Work out the finished part from the listing and answer in its coordinate system (mm). Face numbers are marked on the shaded views. Give positions to 0.01 mm unless a question says otherwise; leave off trailing zeros. Write each loop counter-clockwise with the first axis right and the second up, starting at its lowest first coordinate (ties: lowest second). Pieces come first, ordered by that corner, then holes.
1) Find section C-C (y = -33). Determine the outline of the cut face in (x, z).
2) Given pin 1 Ø3 at (x, y) = (-83.5, -14.5) entering from -Z; pin 2 Ø0.8 at (x, z) = (-30, -0.5) entering from -Y; pin 3 Ø0.5 at (y, z) = (-12.5, -0.5) entering from -X, each flat-ended and moving along its own axis, determine where each tip first touches the part or whether it passes through.
3) Find section A-A (y = -21.5). Determine the outline of the cut face in (x, z), plus the area to 3 significant figures.
4) Find section B-B (x = -116.5). Determine the outline of the cut face in (y, z).
5) Straight lines are drawn through the part: probe 1 along X at (y, z) = (-33, -0.25); probe 2 along Y at (x, z) = (-119.5, 6); probe 3 along Z at (x, y) = (-5, -27). For each, find the intervals that lie inside material, in ascending order.
6) Determine the mould class of the marked faces 1 and 2 for opening direction X: pulls with the +X half, pulls with the -X half, needs draft (parallel to the pull), parting line crosses it, or undercut.
7) Find section D-D (x = -52). Determine the outline of the cut face in (y, z).
```python
from build123d import *

# Parameters (mm, degrees)
SKETCH1_W               = 129.063503861
SKETCH1_H               = 57.862502499
BOSS_EXTRUDE1_DEPTH     = 5
SKETCH2_W               = 36.260872389
SKETCH2_H               = 45.239555314
SKETCH2_W_2             = 34.782772322
SKETCH2_H_2             = 43.550253841
BOSS_EXTRUDE2_DEPTH     = 1
SKETCH3_R               = 3.560103521
BOSS_EXTRUDE3_DEPTH     = 1
CUT_EXTRUDE2_DEPTH      = 0.5
CUT_EXTRUDE3_DEPTH      = 0.5
SKETCH11_W              = 140.269028905
SKETCH11_H              = 63.169878757
BOSS_EXTRUDE4_DEPTH     = 2
CUT_EXTRUDE11_DEPTH     = 146.740563875
CUT_EXTRUDE12_DEPTH     = 149.974025726
CUT_EXTRUDE15_DEPTH     = 149.535595308
CUT_EXTRUDE18_DEPTH     = 149.974025726
CUT_EXTRUDE20_START     = -22.544046022
CUT_EXTRUDE20_OUTLINE_W = 10.649091721
CUT_EXTRUDE20_OUTLINE_H = 19.66096559
CUT_EXTRUDE20_DEPTH     = 22.544046022


# Read off the part's stored shape, not the designer's step: Cut-Extrude20
with BuildPart() as part:
    # Sketch1 → Boss-Extrude1 (new body)
    with BuildSketch(Plane.XY):
        with Locations((-61.962065286, -16.351878859)):
            Rectangle(SKETCH1_W, SKETCH1_H)
    extrude(amount=BOSS_EXTRUDE1_DEPTH)

    # Sketch2 → Boss-Extrude2 (add)
    with BuildSketch(Plane(origin=(0, 0, 0), x_dir=(-1, 0, 0), z_dir=(0, 0, -1))):
        with Locations((32.418116178, -15.92763049)):
            Rectangle(SKETCH2_W, SKETCH2_H)
        with Locations((32.418116178, -15.92763049)):
            Rectangle(SKETCH2_W_2, SKETCH2_H_2, mode=Mode.SUBTRACT)
    extrude(amount=BOSS_EXTRUDE2_DEPTH)

    # Sketch3 → Boss-Extrude3 (add)
    with BuildSketch(Plane(origin=(0, 0, 0), x_dir=(-1, 0, 0), z_dir=(0, 0, -1))):
        with Locations((5.84715491, -15.809376146)):
            Circle(SKETCH3_R)
    extrude(amount=BOSS_EXTRUDE3_DEPTH)

    # Sketch4 → Cut-Extrude2 (cut)
    with BuildSketch(Plane(origin=(0, 0, -1), x_dir=(-1, 0, 0), z_dir=(0, 0, -1))):
        with BuildLine():
            Line((7.498244586, -13.503730374), (7.429945817, -14.22683494))
            ThreePointArc((7.429945817, -14.22683494), (3.750240849, -15.79486572), (7.319195969, -17.600830429))
            Line((7.319195969, -17.600830429), (7.313770936, -18.341402976))
            ThreePointArc((7.313770936, -18.341402976), (3.134365244, -15.759677296), (7.498244586, -13.503730374))
        make_face()
    extrude(amount=-CUT_EXTRUDE2_DEPTH, mode=Mode.SUBTRACT)

    # Sketch5 → Cut-Extrude3 (cut)
    with BuildSketch(Plane(origin=(0, 0, -1), x_dir=(-1, 0, 0), z_dir=(0, 0, -1))):
        with BuildLine():
            Line((8.340052895, -15.49291333), (5.46397868, -15.438165983))
            ThreePointArc((5.46397868, -15.438165983), (5.066360432, -15.835784231), (5.46397868, -16.233402479))
            Line((5.46397868, -16.233402479), (8.340052895, -16.178655131))
            ThreePointArc((8.340052895, -16.178655131), (8.682923796, -15.835784231), (8.340052895, -15.49291333))
        make_face()
    extrude(amount=-CUT_EXTRUDE3_DEPTH, mode=Mode.SUBTRACT)

    # Sketch11 → Boss-Extrude4 (add)
    with BuildSketch(Plane.XY.offset(5)):
        with Locations((-64.601623086, -16.772300036)):
            Rectangle(SKETCH11_W, SKETCH11_H)
    extrude(amount=BOSS_EXTRUDE4_DEPTH)

    # Sketch12 → Cut-Extrude11 (cut, through all)
    with BuildSketch(Plane(origin=(2.569686645, 0, 0), x_dir=(0, 0, -1), z_dir=(1, 0, 0))):
        Polygon((-5.049502584, 12.555506791), (1.376837193, 8.637811028), (1.49491418, 17.884962826), align=None)
    extrude(amount=-CUT_EXTRUDE11_DEPTH, mode=Mode.SUBTRACT)

    # Sketch13 → Cut-Extrude12 (cut, through all)
    with BuildSketch(Plane(origin=(0, 14.812639343, 0), x_dir=(1, 0, 0), z_dir=(0, 1, 0))):
        Polygon((-126.405113906, -5), (-129.311029141, 1.46898876), (-122.374079844, 2.014276014), align=None)
    extrude(amount=-CUT_EXTRUDE12_DEPTH, mode=Mode.SUBTRACT)

    # Sketch14 → Cut-Extrude15 (cut, through all)
    with BuildSketch(Plane.ZY.offset(134.736137539)):
        Polygon((5, -45.234938719), (-1.330755584, -41.178219973), (-1.62330097, -49.506029315), align=None)
    extrude(amount=-CUT_EXTRUDE15_DEPTH, mode=Mode.SUBTRACT)

    # Sketch15 → Cut-Extrude18 (cut, through all)
    with BuildSketch(Plane(origin=(0, -48.357239414, 0), x_dir=(-1, 0, 0), z_dir=(0, -1, 0))):
        Polygon((-2.559600043, -5), (1.778800488, 1.23954643), (-4.071250311, 1.127548689), align=None)
    extrude(amount=-CUT_EXTRUDE18_DEPTH, mode=Mode.SUBTRACT)

    # Cut-Extrude20 outline → Cut-Extrude20 (cut)
    with BuildSketch(Plane(origin=(-92.862199247, 0, -53.366974362), x_dir=(-0.49826909719441087, 0, 0.8670224372996739), z_dir=(-0.8670224372996738, 0, -0.4982690971944108)).offset(CUT_EXTRUDE20_START)):
        with Locations((61.994328313, -17.773281039)):
            Rectangle(CUT_EXTRUDE20_OUTLINE_W, CUT_EXTRUDE20_OUTLINE_H)
    extrude(amount=CUT_EXTRUDE20_DEPTH, mode=Mode.SUBTRACT)


solid = part.part
```
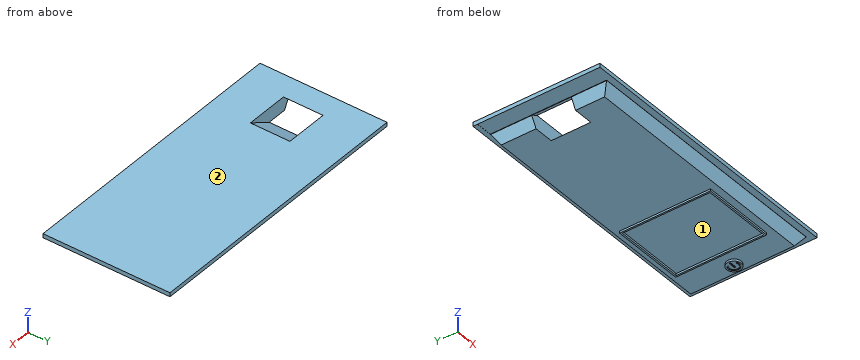
Results:
1. outline: (-134.74, 5) - (-126.49, 5) - (-126.49, 4.8) - (-126.41, 5) - (-123.53, 0) - (-50.55, 0) - (-50.55, -1) - (-49.81, -1) - (-49.81, 0) - (-15.03, 0) - (-15.03, -1) - (-14.29, -1) - (-14.29, 0) - (-0.92, 0) - (2.56, 5) - (2.57, 4.96) - (2.57, 5) - (5.53, 5) - (5.53, 7) - (-134.74, 7) - close
2. pin 1: stops at z = 0
2. pin 2: stops at y = -38.55
2. pin 3: stops at x = -50.55
3. outline: (-134.74, 5) - (-126.49, 5) - (-126.49, 4.8) - (-126.41, 5) - (-122.92, 7) - (-134.74, 7) - close; (-113.73, 0) - (-50.55, 0) - (-50.55, -1) - (-49.81, -1) - (-49.81, 0) - (-15.03, 0) - (-15.03, -1) - (-14.29, -1) - (-14.29, 0) - (-0.92, 0) - (2.56, 5) - (2.57, 4.96) - (2.57, 5) - (5.53, 5) - (5.53, 7) - (-101.55, 7) - close
3. area: 790 mm2
4. outline: (-48.36, 5) - (-45.28, 5) - (-45.28, 4.93) - (-45.23, 5) - (-42.03, 0) - (-27.6, 0) - (-27.6, 7) - (-48.36, 7) - close; (-7.94, 0) - (9.48, 0) - (12.56, 5.05) - (12.6, 5) - (14.81, 5) - (14.81, 7) - (-7.94, 7) - close
5. probe 1: x = -50.55 to -49.81, -15.03 to -14.29
5. probe 2: y = -48.36 to -27.6, -7.94 to 14.81
5. probe 3: z = 0 to 7
6. face 1: undercut
6. face 2: needs draft
7. outline: (-48.36, 5) - (-45.28, 5) - (-45.28, 4.93) - (-45.23, 5) - (-42.03, 0) - (9.48, 0) - (12.56, 5.05) - (12.6, 5) - (14.81, 5) - (14.81, 7) - (-48.36, 7) - close
